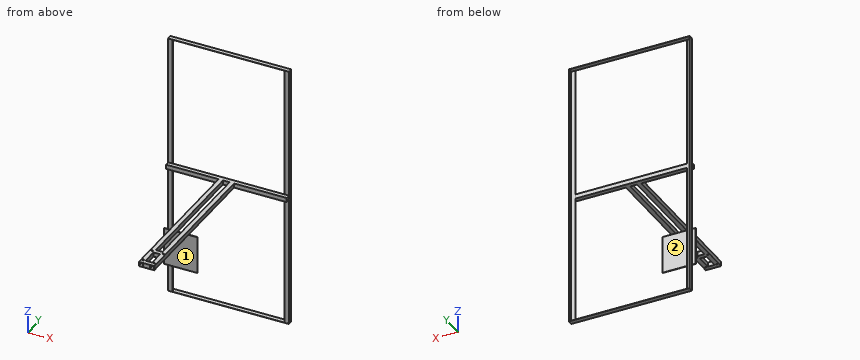
```python
from build123d import *

# Parameters (mm, degrees)
EXTRUDE_THIN1_OUTLINE_W   = 20
EXTRUDE_THIN1_OUTLINE_H   = 20
EXTRUDE_THIN1_OUTLINE_W_2 = 18
EXTRUDE_THIN1_OUTLINE_H_2 = 18
EXTRUDE_THIN1_DEPTH       = 700
EXTRUDE_THIN2_DEPTH       = 238
EXTRUDE_THIN2_DEPTH_BACK  = 308
SKETCH3_W                 = 20
SKETCH3_H                 = 20
SKETCH3_W_2               = 18
SKETCH3_H_2               = 18
F_6_0MM_DOWEL_HOLE1_D     = 6
EXTRUDE_THIN3_DEPTH       = 590
EXTRUDE_THIN3_DEPTH_BACK  = 610
SKETCH8_W                 = 547
SKETCH8_H                 = 21
BOSS_EXTRUDE1_DEPTH       = 1
SKETCH9_W                 = 547
SKETCH9_H                 = 20
BOSS_EXTRUDE4_DEPTH       = 1
SKETCH10_W                = 20
SKETCH10_H                = 20
BOSS_EXTRUDE5_DEPTH       = 30
SKETCH11_W                = 150
SKETCH11_H                = 2
BOSS_EXTRUDE6_DEPTH       = 170


# Read off the part's stored shape, not the designer's step: Extrude-Thin1
with BuildPart() as part:
    # Extrude-Thin1 outline → Extrude-Thin1 (new body)
    # profile 1 of 2: a face of its own
    with BuildSketch(Plane(origin=(0, 0, 0), x_dir=(1, 0, 0), z_dir=(0, 1, 0))):
        with Locations((10, -10)):
            Rectangle(EXTRUDE_THIN1_OUTLINE_W, EXTRUDE_THIN1_OUTLINE_H)
        with Locations((10, -10)):
            Rectangle(EXTRUDE_THIN1_OUTLINE_W_2, EXTRUDE_THIN1_OUTLINE_H_2, mode=Mode.SUBTRACT)
    # profile 2 of 2: a face of its own
    with BuildSketch(Plane(origin=(0, 0, 0), x_dir=(1, 0, 0), z_dir=(0, 1, 0))):
        with Locations((-40, -10)):
            Rectangle(EXTRUDE_THIN1_OUTLINE_W, EXTRUDE_THIN1_OUTLINE_H)
        with Locations((-40, -10)):
            Rectangle(EXTRUDE_THIN1_OUTLINE_W_2, EXTRUDE_THIN1_OUTLINE_H_2, mode=Mode.SUBTRACT)
    extrude(amount=EXTRUDE_THIN1_DEPTH)

    # Sketch3 → Extrude-Thin2 (add, two sides: drawn at the far end of the back side and taken through both)
    with BuildSketch(Plane(origin=(20, 0, 0), x_dir=(0, 0, -1), z_dir=(1, 0, 0)).offset(-EXTRUDE_THIN2_DEPTH_BACK)):
        with Locations((-10, 710)):
            Rectangle(SKETCH3_W, SKETCH3_H)
        with Locations((-10, 710)):
            Rectangle(SKETCH3_W_2, SKETCH3_H_2, mode=Mode.SUBTRACT)
    extrude(amount=EXTRUDE_THIN2_DEPTH + EXTRUDE_THIN2_DEPTH_BACK)

    # 6.0mm Dowel Hole1 (through all)
    with Locations(Plane(origin=(0, 0, 0), x_dir=(-1, 0, 0), z_dir=(0, 0, -1))):
        with Locations((40, 20), (-10, 20), (-10, 100), (40, 100)):
            Hole(F_6_0MM_DOWEL_HOLE1_D / 2)

    # Sketch6 → Extrude-Thin3 (add, two sides: drawn at the far end of the back side and taken through both)
    with BuildSketch(Plane(origin=(0, 0, 0), x_dir=(-1, 0, 0), z_dir=(0, 0, -1)).offset(-EXTRUDE_THIN3_DEPTH_BACK)):
        Polygon((-238, 720), (-258, 720), (-258, 740), (-257, 740), (-257, 721), (-238, 721), align=None)
        Polygon((268, 720), (288, 720), (288, 740), (289, 740), (289, 719), (268, 719), align=None)
    extrude(amount=EXTRUDE_THIN3_DEPTH + EXTRUDE_THIN3_DEPTH_BACK)

    # Sketch8 → Boss-Extrude1 (add)
    with BuildSketch(Plane(origin=(0, 0, -590), x_dir=(-1, 0, 0), z_dir=(0, 0, -1))):
        with Locations((15.5, 729.5)):
            Rectangle(SKETCH8_W, SKETCH8_H)
    extrude(amount=BOSS_EXTRUDE1_DEPTH)

    # Sketch9 → Boss-Extrude4 (add)
    with BuildSketch(Plane.XY.offset(610)):
        with Locations((-15.5, 730)):
            Rectangle(SKETCH9_W, SKETCH9_H)
    extrude(amount=-BOSS_EXTRUDE4_DEPTH)

    # Sketch10 → Boss-Extrude5 (add)
    with BuildSketch(Plane(origin=(-30, 0, 0), x_dir=(0, 0, -1), z_dir=(1, 0, 0))):
        with Locations((-10, 10)):
            Rectangle(SKETCH10_W, SKETCH10_H)
        with Locations((-10, 100)):
            Rectangle(SKETCH10_W, SKETCH10_H)
    extrude(amount=BOSS_EXTRUDE5_DEPTH)

    # Sketch11 → Boss-Extrude6 (add)
    with BuildSketch(Plane(origin=(0, 0, 0), x_dir=(-1, 0, 0), z_dir=(0, 0, -1))):
        with Locations((15, 301)):
            Rectangle(SKETCH11_W, SKETCH11_H)
    extrude(amount=BOSS_EXTRUDE6_DEPTH)


solid = part.part
```
Here's how the part is built. I have some questions about the finished solid (model axes, mm). Face numbers are marked on the shaded views. A direction names the side the tool comes from. Coordinates: 2 decimals unless noted, no trailing zeros. Loops run counter-clockwise (first coordinate to the right, second up) from the corner with the lowest first, then second, coordinate; pieces in that order, holes last. Notation, with made-up numbers: M 79,6 L 121,6 A12 ccw 121,21 Z; hole C -7.75,1.25 d9. An arc over 180 degrees is marked long. One line per item, written item: value.
1. Please list where these lines run through material, in increasing order: probe 1 along Y at (x, z) = (-40, 0.3); probe 2 along Z at (x, y) = (14.5, 52); probe 3 along Y at (x, z) = (53, -141).
Geometry says:
probe 1: y = 0 to 17, 23 to 97, 103 to 720
probe 2: z = 0 to 1, 19 to 20
probe 3: y = 300 to 302
2. Imagine slicing it at C-C (y = 195). List the corners of the cut face in (x, z) for me.
Geometry says:
outline: M -50,0 L -30,0 L -30,20 L -50,20 Z; M 0,0 L 20,0 L 20,20 L 0,20 Z; hole M -49,1 L -31,1 L -31,19 L -49,19 Z; hole M 1,1 L 19,1 L 19,19 L 1,19 Z
3. Imagine slicing it at D-D (z = 129). List the corners of the cut face in (x, y) for me, and give its area (3 significant figures).
Geometry says:
outline: M -289,719 L -268,719 L -268,720 L -288,720 L -288,740 L -289,740 Z; M 238,720 L 258,720 L 258,740 L 257,740 L 257,721 L 238,721 Z
area: 80.0 mm2
4. On a 3-axis mill with a long thin cutter (end or side, diameter ignored), from which of +Z, -Z, +X, -X, +Y, -Y can I reach the whole of each face in a straight line? I mean the marked faces 1 and 2. Say none if no direction works.
Geometry says:
face 1: -Z, +X, -X, -Y
face 2: -Z, +X, -X, +Y
5. Will these pins go through, and if not, where does the flat tip stop? pin 1 Ø9 at (x, y) = (-99, 709) entering from -Z; pin 2 Ø16 at (x, z) = (-18.5, 5) entering from +Y; pin 3 Ø8 at (x, y) = (-40, 20) entering from +Z.
Geometry says:
pin 1: stops at z = 0
pin 2: stops at y = 720
pin 3: stops at z = 20
6. Imagine slicing it at A-A (x = 75.5). List the corners of the cut face in (y, z) for me, and give its area (3 significant figures).
Geometry says:
outline: M 700,0 L 720,0 L 720,20 L 700,20 Z; M 719,-591 L 740,-591 L 740,-590 L 719,-590 Z; M 720,609 L 740,609 L 740,610 L 720,610 Z; hole M 701,1 L 719,1 L 719,19 L 701,19 Z
area: 117 mm2
7. Imagine slicing it at B-B (z = -104). List the corners of the cut face in (x, y) for me, and give its area (3 significant figures).
Geometry says:
outline: M -289,719 L -268,719 L -268,720 L -288,720 L -288,740 L -289,740 Z; M -90,300 L 60,300 L 60,302 L -90,302 Z; M 238,720 L 258,720 L 258,740 L 257,740 L 257,721 L 238,721 Z
area: 380 mm2
